Autodesk Inventor part; units mm, degrees
ref_plane "YZ Plane" through (0, 0, 0) normal (1, 0, 0) x (0, 1, 0)
ref_plane "XZ Plane" through (0, 0, 0) normal (0, 1, 0) x (-1, 0, 0)
ref_plane "XY Plane" through (0, 0, 0) normal (0, 0, 1) x (1, 0, 0)
sketch "Sketch1" plane through (0, 0, 0) normal (0, 1, 0) x (-1, 0, 0)
  line L0 (0, 0) -> (150, 0)
  line L1 (150, 0) -> (150, -250)
  line L2 (150, -250) -> (0, -250)
  line L3 (0, -250) -> (0, 0)
  line L4 (150, -275) -> (150, 0)
  line L5 (75, 0) -> (75, -250) construction
  line L6 (150, 0) -> (400, 0)
  line L7 (400, 0) -> (400, -250)
  line L8 (400, -250) -> (150, -250)
  line L9 (150, -250) -> (150, 0)
  line L10 (150, -250) -> (0, -250)
  line L11 (0, -250) -> (0, -200)
  line L12 (0, -200) -> (150, -200)
  line L13 (150, -200) -> (150, -250)
  line L14 (0, 0) -> (150, 0)
  line L15 (150, 0) -> (150, -50)
  line L16 (150, -50) -> (0, -50)
  line L17 (0, -50) -> (0, 0)
  line L18 (28.5, -180.5) -> (28.5, -69.5)
  line L19 (28.5, -180.5) -> (64.5, -180.5)
  line L20 (64.5, -180.5) -> (64.5, -69.5)
  line L21 (64.5, -69.5) -> (28.5, -69.5)
  line L22 (28.5, -69.5) -> (28.5, -180.5)
  line L23 (46.5, -69.5) -> (46.5, -180.5) construction
  line L24 (64.5, -125) -> (28.5, -125) construction
  circle A0 centre (46.5, -125) radius 1.5
  circle A1 centre (55.5, -80.5) radius 1.5
  circle A2 centre (55.5, -169.5) radius 1.5
  circle A3 centre (37.5, -80.5) radius 1.5
  circle A4 centre (37.5, -169.5) radius 1.5
  line L25 (55.5, -93.25) -> (55.5, -156.75) construction
  line L26 (51.75, -93.25) -> (51.75, -156.75)
  line L27 (59.25, -156.75) -> (59.25, -93.25)
  arc A5 (59.25, -93.25) -> (51.75, -93.25) centre (55.5, -93.25) ccw
  arc A6 (51.75, -156.75) -> (59.25, -156.75) centre (55.5, -156.75) ccw
  line L28 (41.25, -93.25) -> (41.25, -156.75)
  line L29 (33.75, -156.75) -> (33.75, -93.25)
  arc A7 (41.25, -93.25) -> (33.75, -93.25) centre (37.5, -93.25) ccw
  arc A8 (33.75, -156.75) -> (41.25, -156.75) centre (37.5, -156.75) ccw
  line L30 (150, -250) -> (93, -250)
  line L31 (93, -250) -> (93, 0)
  line L32 (93, 0) -> (150, 0)
  line L33 (150, 0) -> (150, -250)
  line L34 (0, -200) -> (93, -200)
  line L35 (93, -200) -> (93, -190.5)
  line L36 (93, -190.5) -> (0, -190.5)
  line L37 (0, -190.5) -> (0, -200)
  line L38 (0, -50) -> (93, -50)
  line L39 (93, -50) -> (93, -59.5)
  line L40 (93, -59.5) -> (0, -59.5)
  line L41 (0, -59.5) -> (0, -50)
  line L42 (377.5, -250) -> (377.5, 0) construction
  line L43 (377.5, -250) -> (337.5, -250) construction
  line L44 (337.5, -250) -> (337.5, -202.5) construction
  line L45 (337.5, -202.5) -> (377.5, -202.5) construction
  line L46 (377.5, -202.5) -> (377.5, -250) construction
  line L47 (377.5, 0) -> (337.5, 0) construction
  line L48 (337.5, 0) -> (337.5, -47.5) construction
  line L49 (337.5, -47.5) -> (377.5, -47.5) construction
  line L50 (377.5, -47.5) -> (377.5, 0) construction
  circle A9 centre (372.5, -242.5) radius 1.75
  circle A10 centre (342.5, -242.5) radius 1.75
  line L51 (377.5, -225) -> (337.5, -225) construction
  line L52 (377.5, -225) -> (417.5, -225) construction
  line L53 (400, -125) -> (150, -125) construction
  circle A11 centre (342.5, -210) radius 1.75
  circle A12 centre (372.5, -210) radius 1.75
  circle A13 centre (372.5, -7.5) radius 1.75
  circle A14 centre (342.5, -7.5) radius 1.75
  circle A15 centre (342.5, -40) radius 1.75
  circle A16 centre (372.5, -40) radius 1.75
  line L54 (400, 0) -> (93, 0)
  line L55 (93, 0) -> (93, 1)
  line L56 (93, 1) -> (400, 1)
  line L57 (400, 1) -> (400, 0)
  line L58 (400, -250) -> (93, -250)
  line L59 (93, -250) -> (93, -251)
  line L60 (93, -251) -> (400, -251)
  line L61 (400, -251) -> (400, -250)
  point P0 (55.5, -125)
  dimension "d0" = 150
  dimension "d1" = 250
  dimension "d9" = 250
  dimension "d10" = 50
  dimension "d11" = 50
  dimension "d14" = 36
  dimension "d15" = 3
  dimension "d16" = 3
  dimension "d18" = 7.5
  dimension "d19" = 57
  dimension "d20" = 9.5
  dimension "d21" = 9.5
  dimension "d22" = 40
  dimension "d23" = 47.5
  dimension "d24" = 40
  dimension "d25" = 47.5
  dimension "d26" = 3.5
  dimension "d27" = 3.5
  dimension "d28" = 180
  dimension "d29" = 3.5
  dimension "d30" = 3.5
  dimension "d166" = 307
  dimension "d167" = 1
  dimension "d168" = 307
  dimension "d169" = 1
extrude "Extrusion1" add sketch "Sketch1" along normal blind 3 contours L55 L56 L57 L6 L0 | L0 L1 L16 L31 | L6 L7 L8 L1 | L16 L1 L12 L31 | L40 L31 L36 L3 | L1 L2 L31 L12 | L61 L60 L4 L8 | L4 L60 L59 L2 | L18 L21 L20 L19
sketch "Sketch9" plane through (0, 3, 0) normal (0, 1, 0) x (1, 0, 0)
  arc A0 (-380, 250) -> (-400, 230) centre (-380, 230) ccw
  arc A1 (-400, 20) -> (-380, 0) centre (-380, 20) ccw
  line L0 (-380, 230) -> (-195, 230) construction
  line L1 (-195, 230) -> (-195, 20) construction
  line L2 (-195, 20) -> (-380, 20) construction
  line L3 (-380, 20) -> (-380, 230) construction
  circle A2 centre (-195, 230) radius 1.5
  circle A3 centre (-195, 20) radius 1.5
  circle A4 centre (-380, 20) radius 1.5
  circle A5 centre (-380, 230) radius 1.5
  line L4 (-287.5, 230) -> (-287.5, 20) construction
  line L5 (-380, 125) -> (-195, 125) construction
  circle A6 centre (-287.5, 230) radius 1.5
  circle A7 centre (-195, 125) radius 1.5
  circle A8 centre (-380, 125) radius 1.5
  circle A9 centre (-287.5, 20) radius 1.5
  point P0 (0, 0)
  dimension "d154" = 185
  dimension "d155" = 210
  dimension "d156" = 3
  dimension "d157" = 3
  dimension "d158" = 3
  dimension "d159" = 3
  dimension "d160" = 3
  dimension "d161" = 3
  dimension "d162" = 3
  dimension "d163" = 3
extrude "Extrusion7" cut sketch "Sketch9" against normal blind 5
fillet "Fillet6" radius 50 2 edges at (-93, 1.5, -190.5) (-93, 1.5, -59.5)
fillet "Fillet7" radius 20 6 edges at (0, 1.5, -59.5) (0, 1.5, -190.5) (-93, 1.5, -251) (-93, 1.5, 1) (-400, 1.5, 1) (-400, 1.5, -251)
properties part number "Chassis Bottom Plate"
Source: CAD feature listing. Evaluate the final solid. Frame: model axes, mm. Give positions to 0.01 mm unless a question says otherwise; leave off trailing zeros. Order: outer loops, then holes, each group sorted by start corner. A loop starts at its lowest first (then second) coordinate and runs counter-clockwise, first axis right, second up.
(1) Contact query for flat-ended pins moving along their axis: P1, Ø3.5, axis at x = -55.5, z = -80.5, coming from the +Y side; P2, Ø1.8, axis at x = -380, z = -230, coming from the +Y side; P3, Ø1.5, axis at y = 2.5, z = -70, coming from the +X side; P4, Ø1.5, axis at x = -37, y = 1, coming from the -Z side. Output: stop coordinate, or through.
(2) Material intervals for line 1 along X through (y, z) = (2.75, -133.5); line 2 along Z through (x, y) = (-342.5, 1.9); line 3 along Z through (x, y) = (-287.5, 1.6), sorted ascending.
(3) Section query A-A (y = 1.75). State how many separate pieces and enclosed holes the cut face has, plus the area to 3 significant figures.
(4) Section query B-B (z = -49). Return the cut outline in (x, y).
(5) Section query C-C (x = -86.5). Return the cut outline in (y, z), plus the area to 3 significant figures.
Outcome:
1. P1: stops at y = 3
1. P2: passes through
1. P3: stops at x = -2.02
1. P4: stops at z = -190.5
2. line 1: x = -400 to -59.25, -51.75 to -41.25, -33.75 to 0
2. line 2: z = -251 to -244.25, -240.75 to -211.75, -208.25 to -41.75, -38.25 to -9.25, -5.75 to 1
2. line 3: z = -251 to -231.5, -228.5 to -21.5, -18.5 to 1
3. separate pieces: 1
3. enclosed holes: 23
3. area: 88,900 mm2
4. outline: (-400, 0) - (-73.66, 0) - (-73.66, 3) - (-400, 3) - close
5. outline: (0, -215.85) - (3, -215.85) - (3, -34.15) - (0, -34.15) - close
5. area: 545 mm2
